Here's how the part is built. I have some questions about the finished solid (model axes, mm). Face numbers are marked on the shaded views. Round coordinates to 2 decimals unless told otherwise and drop trailing zeros. Loops run counter-clockwise (first coordinate to the right, second up) from the corner with the lowest first, then second, coordinate; pieces in that order, holes last. Notation, with made-up numbers: M 89.25,-30 L 142.25,-30 A18 ccw 142.25,-1 Z; hole C 27,50 d3. An arc over 180 degrees is marked long. Answer as CSV lines item,"result".
```python
from build123d import *

# Parameters (mm, degrees)
SKETCH_1_R      = 8.5
EXTRUDE_1_DEPTH = 3
FILLET_1_R      = 1


with BuildPart() as part:
    # 草图1 → 凸台-拉伸1 (new body)
    with BuildSketch(Plane(origin=(0, 0, 0), x_dir=(1, 0, 0), z_dir=(0, 1, 0))):
        Polygon((0, 13.856406461), (-12, 6.92820323), (-12, -6.92820323), (0, -13.856406461), (12, -6.92820323), (12, 6.92820323), align=None)
        with Locations(Location((0, 0, 0), (0, 0, 270))):
            Circle(SKETCH_1_R, mode=Mode.SUBTRACT)
    extrude(amount=EXTRUDE_1_DEPTH)

    # 圆角1
    fillet_1_edges = [part.edges().sort_by_distance(p)[0] for p in [
        (-12, 3, 0),
        (-6, 3, 10.392304845),
        (6, 3, 10.392304845),
        (0, 3, -8.5),
        (12, 3, 0),
        (6, 3, -10.392304845),
        (-6, 3, -10.392304845),
    ]]
    fillet(fillet_1_edges, radius=FILLET_1_R)


solid = part.part
```
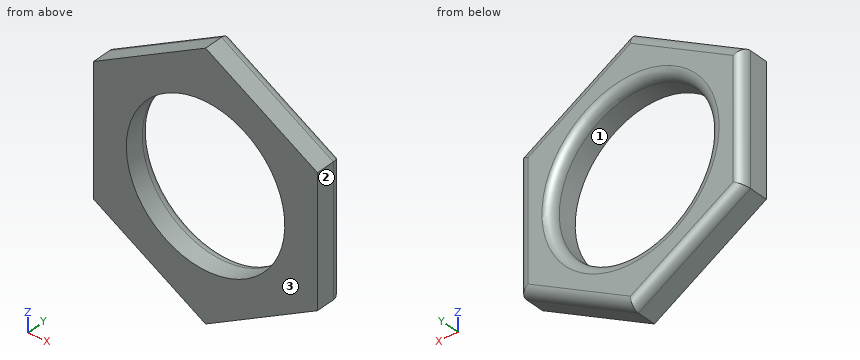
1. We'd pull the mould along X, two halves only. Please class the marked faces 1, 2 and 3: pulls with the +X half, pulls with the -X half, needs draft (parallel to the pull), parting line crosses it, or undercut.
Evaluation:
face 1,"undercut"
face 2,"pulls with the +X half"
face 3,"needs draft"
2. I want a section at B-B, the plane y = 1.15. Please give me the cut outline in (x, z), and give its area (3 significant figures).
Evaluation:
outline,"M -12,-6.93 L 0,-13.86 L 12,-6.93 L 12,6.93 L 0,13.86 L -12,6.93 Z; hole C 0,0 d17"
area,"272 mm²"
3. I want a section at A-A, the plane z = 0. Please give me the cut outline in (x, y).
Evaluation:
outline,"M -12,0 L -8.5,0 L -8.5,2 A1 ccw -9.5,3 L -11,3 A1 ccw -12,2 Z; M 8.5,0 L 12,0 L 12,2 A1 ccw 11,3 L 9.5,3 A1 ccw 8.5,2 Z"
4. For P1, Ø13.5, axis at x = 0, z = 0, coming from the +Y side, with a flat end and sliding along its axis, tell me the tip position at first contact or that it passes through.
Evaluation:
P1,"passes through"
5. If I drill on line 1 (X direction, y = 0.85, z = 0); line 2 (X direction, y = 0.9, z = 6.5); line 3 (Z direction, x = 2, y = 2.1), over which ranges is the centre line in solid material (lowest first)? Write a range as [from, to].
Evaluation:
line 1,"x = [-12, -8.5], [8.5, 12]"
line 2,"x = [-12, -5.48], [5.48, 12]"
line 3,"z = [-12.7, -8.27], [8.27, 12.7]"
